The model under review builds one solid part; all positions refer to its coordinate system, in mm. Face numbers are marked on the shaded views. Coordinates: 2 decimals unless noted, no trailing zeros. Order: outer loops, then holes, each group sorted by start corner. A loop starts at its lowest first (then second) coordinate and runs counter-clockwise, first axis right, second up. Notation, with made-up numbers: M 32.5,40 L 36.5,40 A18 ccw 36.5,70 Z; hole C 63,77.25 d3. An arc over 180 degrees is marked long. Answer as CSV lines item,"result". Start each with the question number.
Q1. Consider section B-B on x = 42. Write out the cut boundary in (y, z), and give its area (3 significant figures).
Q2. For P1, Ø1, axis at y = 70.5, z = 102.5, coming from the +X side; P2, Ø10, axis at y = -36, z = 35.5, coming from the -X side; P3, Ø1, axis at y = -64.5, z = 129.5, coming from the -X side, all flat-tipped, find the tip position at first contact; note any pin that passes through.
Q3. The part is to be moulded in two halves that separate along Y. For the marked faces 1 and 2, say which applies: +Y half, -Y half, draft (parallel to the pull), parting line (faces both ways), or undercut.
Q4. Wall thickness on L1, parallel to Y at x = 0, z = 75.5; L2, parallel to X at y = -2, z = 66.5; L3, parallel to X at y = 23, z = 112: over which ranges is each line inside the solid? List them lowest first. Write a range as [from, to].
Q5. Consider section C-C on z = 63. Write out the cut boundary in (x, y), and give its area (3 significant figures).
Q6. Consider section A-A on y = 0. Write out the cut boundary in (x, z).
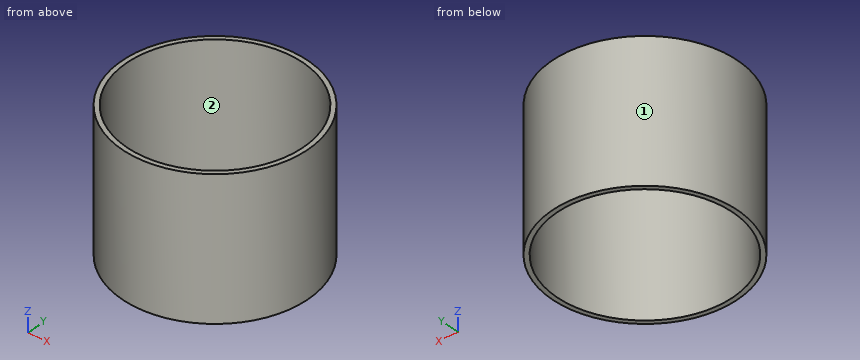
from build123d import *

# Parameters (mm, degrees)
SKETCH1_R           = 100
BOSS_EXTRUDE1_DEPTH = 160
SKETCH2_R           = 95
CUT_EXTRUDE1_DEPTH  = 150
SKETCH3_R           = 10
CUT_EXTRUDE2_DEPTH  = 150
CUT_EXTRUDE4_START  = -10
SKETCH8_R           = 100
CUT_EXTRUDE4_DEPTH  = 10


with BuildPart() as part:
    # Sketch1 → Boss-Extrude1 (new body)
    with BuildSketch(Plane.XY):
        Circle(SKETCH1_R)
    extrude(amount=BOSS_EXTRUDE1_DEPTH)

    # Sketch2 → Cut-Extrude1 (cut)
    with BuildSketch(Plane(origin=(0, 0, 0), x_dir=(-1, 0, 0), z_dir=(0, 0, -1))):
        Circle(SKETCH2_R)
    extrude(amount=-CUT_EXTRUDE1_DEPTH, mode=Mode.SUBTRACT)

    # Sketch3 → Cut-Extrude2 (cut)
    with BuildSketch(Plane.XY.offset(160)):
        Circle(SKETCH3_R)
    extrude(amount=-CUT_EXTRUDE2_DEPTH, mode=Mode.SUBTRACT)

    # Sketch8 → Cut-Extrude4 (cut)
    with BuildSketch(Plane.XY.offset(160).offset(CUT_EXTRUDE4_START)):
        Circle(SKETCH8_R)
    extrude(amount=CUT_EXTRUDE4_DEPTH, mode=Mode.SUBTRACT)


solid = part.part
Evaluation:
1,outline,"M -90.75,0 L -85.21,0 L -85.21,150 L -90.75,150 Z; M 85.21,0 L 90.75,0 L 90.75,150 L 85.21,150 Z"
1,area,"1,660 mm²"
2,P1,"stops at x = 71.41"
2,P2,"stops at x = -95.07"
2,P3,"stops at x = -76.84"
3,face 1,"parting line"
3,face 2,"undercut"
4,L1,"y = [-100, -95], [95, 100]"
4,L2,"x = [-99.98, -94.98], [94.98, 99.98]"
4,L3,"x = [-97.32, -92.17], [92.17, 97.32]"
5,outline,"C 0,0 d200; hole C 0,0 d190"
5,area,"3,060 mm²"
6,outline,"M -100,0 L -95,0 L -95,150 L -100,150 Z; M 95,0 L 100,0 L 100,150 L 95,150 Z"
